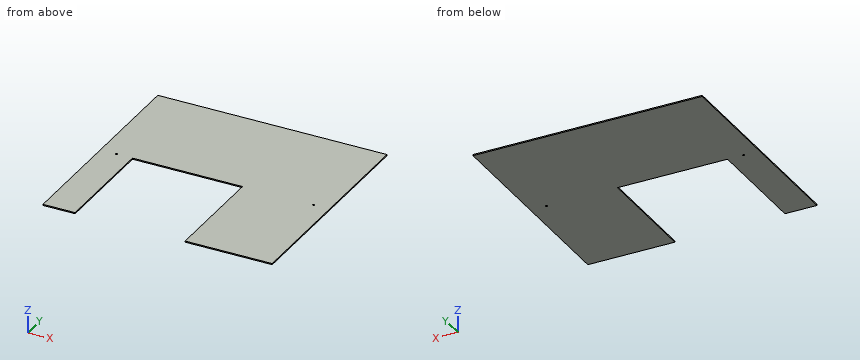
from build123d import *

# Parameters (mm, degrees)
BOSS_EXTRUDE1_DEPTH = 3.175
SKETCH2_R           = 2.5796875
CUT_EXTRUDE1_DEPTH  = 3.175


with BuildPart() as part:
    # Sketch1 → Boss-Extrude1 (new body)
    with BuildSketch(Plane.XY):
        Polygon((-630.182303707, 436.398885794), (4.817696293, 436.398885794), (4.817696293, -173.201114206), (-236.482303707, -173.201114206), (-236.482303707, 131.598885794), (-541.282303707, 131.598885794), (-541.282303707, -173.201114206), (-630.182303707, -173.201114206), align=None)
    extrude(amount=BOSS_EXTRUDE1_DEPTH)

    # Sketch2 → Cut-Extrude1 (cut)
    with BuildSketch(Plane.XY.offset(3.175)):
        with Locations((-585.732303707, 131.598885794)):
            Circle(SKETCH2_R)
        with Locations((-39.632303707, 131.598885794)):
            Circle(SKETCH2_R)
    extrude(amount=-CUT_EXTRUDE1_DEPTH, mode=Mode.SUBTRACT)


solid = part.part
Model file for the job. Use its own axes, mm. Give positions to 0.01 mm unless a question says otherwise; leave off trailing zeros. Loops run counter-clockwise (first coordinate to the right, second up) from the corner with the lowest first, then second, coordinate; pieces in that order, holes last. Notation, with made-up numbers: (33.5, 20) -> (78.5, 20) arc R22 cw to (78.5, 37) -> close; hole circle Ø4 at (87.5, 45). An arc over 180 degrees is marked (long way). Use a Markdown table: item, result. Add a question column.
(1) Wall check: line 1 along X through (y, z) = (103.5, 1.35); line 2 along Y through (x, z) = (-536, 2.15). Give the ranges that are in metal, low to high.
(2) Slice it at A-A on y = 95. List the corners of the cut face in (x, z) (3 decimals).
(3) Drop a flat-ended pin along its axis: pin 1 Ø1.6 at (x, z) = (-446, 1) entering from -Y. Give the stop position or say it passes through.
(4) Slice it at B-B on z = 1.45. List the corners of the cut face in (x, y), and give its area (3 significant figures).
(5) Slice it at C-C on x = -451. List the corners of the cut face in (y, z) (3 decimals), and give its area (3 significant figures).
Filled sheet:
| question | item | result |
|---|---|---|
| 1 | line 1 | -630.18 to -541.28, -236.48 to 4.82 |
| 1 | line 2 | 131.6 to 436.4 |
| 2 | outline | (-630.182, 0) -> (-541.282, 0) -> (-541.282, 3.175) -> (-630.182, 3.175) -> close; (-236.482, 0) -> (4.818, 0) -> (4.818, 3.175) -> (-236.482, 3.175) -> close |
| 3 | pin 1 | y = 131.6 |
| 4 | outline | (-630.18, -173.2) -> (-541.28, -173.2) -> (-541.28, 131.6) -> (-236.48, 131.6) -> (-236.48, -173.2) -> (4.82, -173.2) -> (4.82, 436.4) -> (-630.18, 436.4) -> close; hole circle Ø5.16 at (-585.73, 131.6); hole circle Ø5.16 at (-39.63, 131.6) |
| 4 | area | 294,000 mm2 |
| 5 | outline | (131.599, 0) -> (436.399, 0) -> (436.399, 3.175) -> (131.599, 3.175) -> close |
| 5 | area | 968 mm2 |
